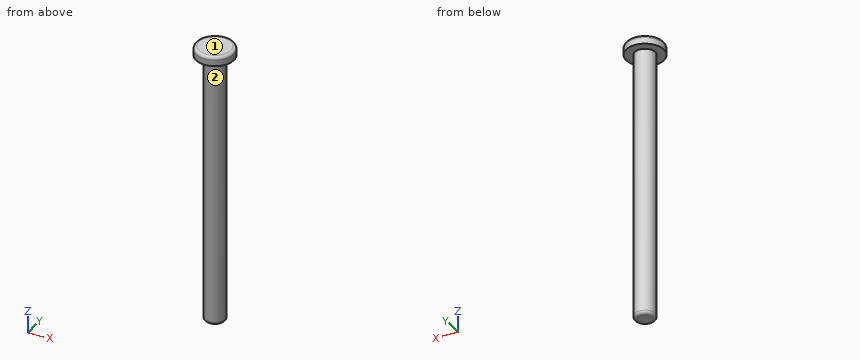
Solid Edge part; units mm, degrees
sketch "Sketch1" plane through (0, 0, 0) normal (0, 0, 1) x (1, 0, 0)
  circle A0 centre (0, 0) radius 3.3483
extrude "Protrusion1" add sketch "Sketch1" against normal up to vertex (88.9 mm away)
fillet "Round1" radius 1 1 edges at (-3.3483, 0, -88.9)
sketch "Sketch2" plane through (0, 0, 0) normal (0, 0, 1) x (0, -1, 0)
  circle A0 centre (0, 0) radius 6.1767
extrude "ExtrudedProtrusion_2" add sketch "Sketch2" along normal blind 3
fillet "Round_2" radius 1 1 edges at (0, 6.1767, 3)
Geometry check sheet. Reference: the model listing, model coordinates, mm. Face numbers are marked on the shaded views. Coordinates: 2 decimals unless noted, no trailing zeros. Loops run counter-clockwise (first coordinate to the right, second up) from the corner with the lowest first, then second, coordinate; pieces in that order, holes last. Notation, with made-up numbers: (38, 18.5) - (86, 18.5) arc R11 ccw to (86, 37.5) - close; hole circle Ø6 at (-39, -15.75). An arc over 180 degrees is marked (long way). One line per item, written item: value. Start each with the question number.
(1) Depth check by flat-ended pin: P1, Ø2, axis at x = -0.5, y = 2.5, coming from the -Z side; P2, Ø1.5, axis at x = 3, y = 2, coming from the -Z side; P3, Ø1.5, axis at x = 3, z = -15.5, coming from the -Y side. Enter the tip coordinate at first touch or a pass-through.
(2) Material ranges on line 1 (Z direction, x = -2, y = -3.25); line 2 (Z direction, x = 4.25, y = 3.75); line 3 (Y direction, x = 2, z = -66), recorded low to high. Write a range as [from, to].
(3) Mould release check, pull along Z, two halves, no side actions. Record for the marked faces 1 and 2: released by +Z, released by -Z, zero draft, split by the parting line, or undercut.
(4) Cross-section at A-A on y = 0. Enter the section's corners in (x, z).
(5) Cross-section at C-C on z = -70. Enter the section's corners in (x, y), plus the area to 3 significant figures.
Results below:
1. P1: stops at z = -88.9
1. P2: stops at z = -88.76
1. P3: stops at y = -2.48
2. line 1: z = [0, 3]
2. line 2: z = [0, 2.87]
2. line 3: y = [-2.69, 2.69]
3. face 1: released by +Z
3. face 2: zero draft
4. outline: (-6.18, 0) - (-3.35, 0) - (-3.35, -87.9) arc R1 ccw to (-2.35, -88.9) - (2.35, -88.9) arc R1 ccw to (3.35, -87.9) - (3.35, 0) - (6.18, 0) - (6.18, 2) arc R1 ccw to (5.18, 3) - (-5.18, 3) arc R1 ccw to (-6.18, 2) - close
5. outline: circle Ø6.7 at (0, 0)
5. area: 35.2 mm2
